```python
from build123d import *

# Parameters (mm, degrees)
BOSS_EXTRUDE2_DEPTH = 1
SKETCH2_R           = 2
CUT_EXTRUDE1_DEPTH  = 52.686248125
BOSS_EXTRUDE3_DEPTH = 0.5
CUT_EXTRUDE3_START  = -2
CUT_EXTRUDE3_DEPTH  = 2
FILLET1_R           = 5
FILLET2_R           = 0.5


# Read off the part's stored shape, not the designer's step: Cut-Extrude3
with BuildPart() as part:
    # Sketch1 → Boss-Extrude2 (new, symmetric)
    with BuildSketch(Plane(origin=(0, 0, 0), x_dir=(1, 0, 0), z_dir=(0, 1, 0))):
        with BuildLine():
            Line((48.296291314, -12.940952255), (0, 0))
            Line((0, 0), (48.296291314, 12.940952255))
            ThreePointArc((48.296291314, 12.940952255), (50, 0), (48.296291314, -12.940952255))
        make_face()
    extrude(amount=BOSS_EXTRUDE2_DEPTH, both=True)

    # Sketch2 → Cut-Extrude1 (cut, through all)
    with BuildSketch(Plane(origin=(0, 1, 0), x_dir=(1, 0, 0), z_dir=(0, 1, 0))):
        with Locations(Location((42.5, 0, 0), (0, 0, 270))):
            Circle(SKETCH2_R)
    extrude(amount=-CUT_EXTRUDE1_DEPTH, mode=Mode.SUBTRACT)

    # Sketch3 → Boss-Extrude3 (add)
    with BuildSketch(Plane(origin=(0, -1, 0), x_dir=(-1, 0, 0), z_dir=(0, -1, 0))):
        with BuildLine():
            Line((-38.5, -7), (-38.5, 7))
            ThreePointArc((-38.5, 7), (-38, 7.5), (-37.5, 7))
            Line((-37.5, 7), (-37.5, -7))
            ThreePointArc((-37.5, -7), (-38, -7.5), (-38.5, -7))
        make_face()
    extrude(amount=BOSS_EXTRUDE3_DEPTH)

    # Cut-Extrude3 outline → Cut-Extrude3 (cut)
    with BuildSketch(Plane(origin=(0, 1, 0), x_dir=(1, 0, 0), z_dir=(0, 1, 0)).offset(CUT_EXTRUDE3_START)):
        with BuildLine():
            ThreePointArc((39.129720832, 10.484777097), (44.969397941, 4.720942194), (49.96810207, -1.785714286))
            ThreePointArc((49.96810207, -1.785714286), (49.680896013, 5.639908806), (48.296291314, 12.940952255))
            Line((48.296291314, 12.940952255), (39.129720832, 10.484777097))
        make_face()
    extrude(amount=CUT_EXTRUDE3_DEPTH, mode=Mode.SUBTRACT)

    # Fillet1
    fillet1_edges = [part.edges().sort_by_distance(p)[0] for p in [
        (39.129720832, 0, -10.484777097),
        (49.96810207, 0, 1.785714286),
        (48.296291314, 0, 12.940952255),
    ]]
    fillet(fillet1_edges, radius=FILLET1_R)

    # Fillet2
    fillet2_edges = [part.edges().sort_by_distance(p)[0] for p in [
        (18.252899917, -1, -4.890849792),
        (18.252899917, 1, -4.890849792),
        (45.320316883, -1, -4.32008237),
        (49.692435611, -1, 5.537313704),
        (21.598758088, -1, 5.787369787),
        (47.228674266, -1, 10.929424828),
        (49.700770587, -1, 1.869330184),
        (39.027043508, -1, -9.799142423),
        (45.320316883, 1, -4.32008237),
        (21.598758088, 1, 5.787369787),
        (49.692435611, 1, 5.537313704),
        (47.228674266, 1, 10.929424828),
        (49.700770587, 1, 1.869330184),
        (39.027043508, 1, -9.799142423),
    ]]
    fillet(fillet2_edges, radius=FILLET2_R)


solid = part.part
```
Model file for the job. Use its own axes, mm. Give positions to 0.01 mm unless a question says otherwise; leave off trailing zeros. Write each question's results on one line, items separated by ' | '.
(1) Probe line 1 along Y through (x, z) = (18.5, -3); line 2 along X through (y, z) = (-1.3, 4.5); line 3 along Z through (x, y) = (8.5, 0.6). List the from-to ranges inside material, lowest first.
Geometry results:
line 1: y = -1 to 1 | line 2: x = 37.5 to 38.5 | line 3: z = -2.27 to 2.27
(2) Pull direction X, two halves, no side cores. Call faces 1 (the cylindrical face through (49.695, 0.007, 5.51)), 2 (the cylindrical face through (40.548, 0.014, -0.434)), 3 (the cylindrical face through (18.55, -0.86, -4.81)): released by +X, released by -X, zero draft, split by the parting line, or undercut.
Geometry results:
face 1: released by +X | face 2: undercut | face 3: released by -X
(3) Flat gauge pins, fed straight in: pin 1 Ø0.6 at (y, z) = (-1.5, -0.5) entering from -X; pin 2 Ø6.5 at (x, z) = (42.5, 0) entering from +Y; pin 3 Ø1.5 at (x, y) = (39, -1) entering from -Z; pin 4 Ø6 at (x, z) = (27.5, -0.5) entering from -Y. Where does each tip first touch, or does it go through?
Geometry results:
pin 1: stops at x = 37.5 | pin 2: stops at y = 1 | pin 3: stops at z = -9.91 | pin 4: stops at y = -1
